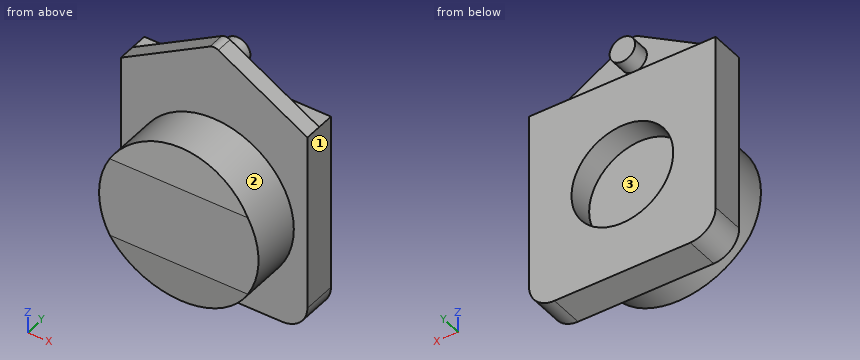
Autodesk Inventor part; units mm, degrees
ref_plane "작업 평면1" through (0, 50, 0) normal (0, 1, 0) x (1, 0, 0)
ref_plane "YZ Plane" through (0, 0, 0) normal (1, 0, 0) x (0, 1, 0)
ref_plane "XZ Plane" through (0, 0, 0) normal (0, 1, 0) x (-1, 0, 0)
sketch "스케치1" plane through (0, 0, 0) normal (0, 1, 0) x (-1, 0, 0)
  circle A0 centre (0, 0) radius 47
  circle A1 centre (0, 0) radius 35
  line L0 (0, 0) -> (0, 145.5)
  circle A2 centre (0, 145.5) radius 48.5
  circle A3 centre (0, 145.5) radius 36.5
  dimension "d0" = 94
  dimension "d1" = 12
  dimension "d2" = 145.5
  dimension "d3" = 97
  dimension "d4" = 12
extrude "돌출1" add sketch "스케치1" along normal blind 30 contours A0
sketch "스케치2" plane through (0, 30, 0) normal (0, 1, 0) x (1, 0, 0)
  line L0 (-55, 60) -> (55, 60)
  line L1 (55, 60) -> (55, -60)
  line L2 (55, -60) -> (-55, -60)
  line L3 (-55, -60) -> (-55, 60)
  line L4 (-55, 60) -> (55, -60) construction
  line L5 (55, 60) -> (-55, -60) construction
  point P0 (0, 0)
  dimension "d7" = 110
  dimension "d8" = 120
extrude "돌출2" add sketch "스케치2" along normal blind 20
sketch "스케치3" plane through (0, 30, 0) normal (0, -1, 0) x (1, 0, 0)
  line L0 (-55, 60) -> (55, 60)
  line L1 (-55, 60) -> (0, 91.7543)
  line L2 (-55, 60) -> (8.5085, 60) construction
  line L3 (0, 91.7543) -> (55, 60)
  line L4 (55, 60) -> (-55, 60)
  line L5 (0, 91.7543) -> (0, 76.7543)
  circle A0 centre (0, 76.7543) radius 7.5
  point P0 (0, 0)
  dimension "d11" = 30
  dimension "d12" = 15
  dimension "d13" = 15
  dimension "d20" = 30
extrude "돌출3" add sketch "스케치3" against normal blind 10 contours L1 L3 L0 | A0
sketch "스케치4" plane through (0, 40, 0) normal (0, 1, 0) x (1, 0, 0)
  line L0 (55, -60) -> (0, -91.7543)
  line L1 (0, -91.7543) -> (0, -76.7543)
  circle A0 centre (0, -76.7543) radius 7.5
  point P0 (0, 0)
  dimension "d16" = 15
  dimension "d17" = 15
extrude "돌출4" add sketch "스케치4" along normal blind 10
fillet "모깎기1" radius 15 2 edges at (-55, 40, -60) (55, 40, -60)
ref_plane "작업 평면1" through (0, 50, 0) normal (0, 1, 0) x (1, 0, 0)
sketch "스케치6" plane through (0, 50, 0) normal (0, 1, 0) x (1, 0, 0)
  circle A0 centre (0, 0) radius 30
extrude "돌출6" cut sketch "스케치6" against normal blind 15
fillet "모깎기2" radius 5 1 edges at (0, 35, 91.7543)
sketch "스케치7" plane through (0, 0, 0) normal (0, -1, 0) x (1, 0, 0)
  circle A0 centre (0, 0) radius 35
extrude "돌출7" add sketch "스케치7" against normal up to surface (30 mm away)
sketch "스케치8" plane through (0, 0, 0) normal (1, 0, 0) x (0, 1, 0)
  line L0 (0, -47) -> (0, 47)
  line L1 (0, 0) -> (0, 47)
  line L2 (0, 23.5) -> (2.056, 47)
  line L3 (0, 47) -> (30, 47)
  line L4 (0, 23.5) -> (23.5898, 23.5) construction
  line L5 (2.056, 47) -> (0, 47)
  line L6 (0, 0) -> (0, -47)
  line L7 (0, -23.5) -> (0, -47)
  line L8 (0, -47) -> (30, -47)
  line L9 (0, -47) -> (0, -47)
  line L10 (0, -23.5) -> (0, -47)
  line L11 (0, -47) -> (0, -47)
  line L12 (0, -23.5) -> (2.056, -47)
  line L13 (0, -23.5) -> (23.5898, -23.5) construction
  line L14 (2.056, -47) -> (0, -47)
  dimension "d31" = 85
  dimension "d32" = 85
extrude "돌출8" cut sketch "스케치8" along normal mid plane 100
properties part number "bracket_1"
Design review of the part built by this model. Coordinates are the model's own, in mm. Face numbers are marked on the shaded views. A direction names the side the tool comes from. Round coordinates to 2 decimals unless told otherwise and drop trailing zeros. Write each loop counter-clockwise with the first axis right and the second up, starting at its lowest first coordinate (ties: lowest second). Pieces come first, ordered by that corner, then holes. Notation, with made-up numbers: (47, -4) - (63, -4) arc R12 ccw to (63, 16) - close; hole circle Ø4 at (-14.5, 81.25). An arc over 180 degrees is marked (long way). Use a Markdown table: item, result. Add a question column.
1. Wall thickness on probe 1 along Z at (x, y) = (0, 41); probe 2 along X at (y, z) = (39.25, 0); probe 3 along Z at (x, y) = (0, 39.75): over which ranges is each line inside the solid? List them lowest first.
2. We need section A-A (z = 0). State the section outline as (x, y) points, then the cut area to 3 significant figures.
3. For the marked faces 1, 2 and 3, list the 3-axis set-ups (+Z, -Z, +X, -X, +Y, -Y) from which the entire face can be reached by the end or side of a thin tool; tool diameter is ignored.
4. We need section B-B (x = 0). State the section outline as (y, z) points.
5. We need section D-D (z = 71). State the section outline as (x, y) points, then the cut area to 3 significant figures.
6. We need section C-C (y = 17). State the section outline as (x, z) points.
7. Clearance check with flat-ended pins moving along their axes: pin 1 (1 mm diameter, centred on y = 14, z = -21.5, fed in from -X); pin 2 (2 mm diameter, centred on x = 14, y = 37.5, fed in from +Z); pin 3 (12 mm diameter, centred on x = -32, y = 15, fed in from +Z). State where each tip first meets the part, or that it passes through.
Output:
| question | item | result |
|---|---|---|
| 1 | probe 1 | z = -60 to -30, 30 to 60, 69.25 to 84.25 |
| 1 | probe 2 | x = -55 to -30, 30 to 55 |
| 1 | probe 3 | z = -60 to -30, 30 to 90.98 |
| 2 | outline | (-55, 30) - (-47, 30) - (-47, 0) - (47, 0) - (47, 30) - (55, 30) - (55, 50) - (30, 50) - (30, 35) - (-30, 35) - (-30, 50) - (-55, 50) - close |
| 2 | area | 4,120 mm2 |
| 3 | face 1 | +Z, -Z, +X, +Y, -Y |
| 3 | face 2 | -Y |
| 3 | face 3 | +Y |
| 4 | outline | (0, -23.5) - (2.06, -47) - (30, -47) - (30, -60) - (50, -60) - (50, -30) - (35, -30) - (35, 30) - (50, 30) - (50, 60) - (40, 60) - (40, 69.25) - (50, 69.25) - (50, 84.25) - (40, 84.25) - (40, 90.98) - (30, 90.98) - (30, 47) - (2.06, 47) - (0, 23.5) - close |
| 5 | outline | (-35.95, 30) - (35.95, 30) - (35.95, 40) - (4.81, 40) - (4.81, 50) - (-4.81, 50) - (-4.81, 40) - (-35.95, 40) - close |
| 5 | area | 815 mm2 |
| 6 | outline | circle Ø94 at (0, 0) |
| 7 | pin 1 | stops at x = -42.05 |
| 7 | pin 2 | stops at z = 84.25 |
| 7 | pin 3 | stops at z = 39.15 |
